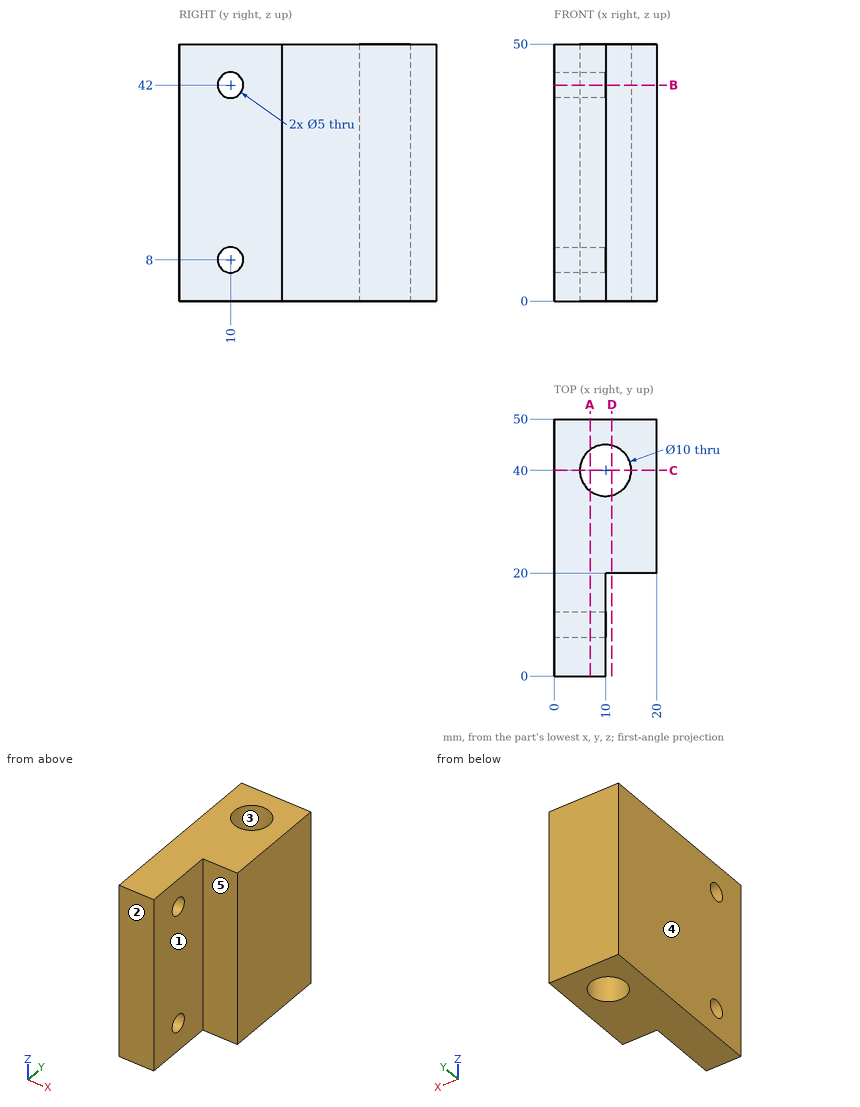
Geometry check sheet. Reference: drawing and pictorial views, mm from the part's lowest x, y, z. A direction names the side the tool comes from. Round coordinates to 2 decimals unless told otherwise and drop trailing zeros. Loops run counter-clockwise (first coordinate to the right, second up) from the corner with the lowest first, then second, coordinate; pieces in that order, holes last. Notation, with made-up numbers: (79.5, -1) -> (123.5, -1) arc R23 cw to (123.5, 15) -> close; hole circle Ø9 at (49.5, -13). An arc over 180 degrees is marked (long way). Answer as a JSON object with one key per item and string values.
Q1. Section check C-C (y = 40). Record the boundary of the cut face in (x, z).
Data:
{"outline": "(0, 0) -> (5, 0) -> (5, 50) -> (0, 50) -> close; (15, 0) -> (20, 0) -> (20, 50) -> (15, 50) -> close"}
Q2. Draft check along Y on the marked faces 1, 2 and 3. Enter one of: pulls with the +Y half, pulls with the -Y half, needs draft (parallel to the pull), parting line crosses it, or undercut.
Data:
{"face 1": "needs draft", "face 2": "pulls with the -Y half", "face 3": "undercut"}
Q3. Scan lines: line 1 (X direction, y = 13.5, z = 7.5); line 2 (Y direction, x = 16.25, z = 3); line 3 (Y direction, x = 4, z = 8). Record each from-to range of solid material in increasing order. Write a range as from..to.
Data:
{"line 1": "x = 0..10", "line 2": "y = 20..50", "line 3": "y = 0..7.5, 12.5..50"}
Q4. Go/stop test with flat-tipped pins: P1, Ø9, axis at x = 10, y = 40, coming from the -Z side; P2, Ø8, axis at y = 10.5, z = 43.5, coming from the +X side. Record where each tip stops, or that it passes through.
Data:
{"P1": "passes through", "P2": "stops at x = 10"}
Q5. Section check B-B (z = 42). Record the boundary of the cut face in (x, y).
Data:
{"outline": "(0, 0) -> (10, 0) -> (10, 7.5) -> (0, 7.5) -> close; (0, 12.5) -> (10, 12.5) -> (10, 20) -> (20, 20) -> (20, 50) -> (0, 50) -> close; hole circle Ø10 at (10, 40)"}
Q6. Section check D-D (x = 11.25). Record the boundary of the cut face in (y, z), then the cut area to 3 significant figures.
Data:
{"outline": "(20, 0) -> (35.16, 0) -> (35.16, 50) -> (20, 50) -> close; (44.84, 0) -> (50, 0) -> (50, 50) -> (44.84, 50) -> close", "area": "1,020 mm2"}
Q7. Section check A-A (x = 7). Record the boundary of the cut face in (y, z), then the cut area to 3 significant figures.
Data:
{"outline": "(0, 0) -> (36, 0) -> (36, 50) -> (0, 50) -> close; (44, 0) -> (50, 0) -> (50, 50) -> (44, 50) -> close; hole circle Ø5 at (10, 8); hole circle Ø5 at (10, 42)", "area": "2,060 mm2"}
Q8. Access from +Z, -Z, +X, -X, +Y, -Y to the whole of each face (thin tool, end or side, straight path). Record for the marked faces 4 and 5.
Data:
{"face 4": "+Z, -Z, -X, +Y, -Y", "face 5": "+Z, -Z, +X, -Y"}
